from build123d import *

# Parameters (mm, degrees)
BOSS_EXTRUDE1_START     = -2.5
BOSS_EXTRUDE1_DEPTH     = 26.5
CUT_EXTRUDE1_START      = -3
CUT_EXTRUDE1_DEPTH      = 25.6
CUT_EXTRUDE2_DEPTH      = 53.459508194
CUT_EXTRUDE2_DEPTH_BACK = 53.459508194
SKETCH3_W               = 33
SKETCH3_H               = 5.5
CUT_EXTRUDE3_DEPTH      = 53.459508194
CUT_EXTRUDE3_DEPTH_BACK = 53.459508194
SKETCH4_R               = 1.2


with BuildPart() as part:
    # Sketch1 → Boss-Extrude1 (new body)
    with BuildSketch(Plane.XY.offset(BOSS_EXTRUDE1_START)):
        Polygon((40, 16), (39.846282243, 17.560722576), (39.39103626, 19.061467459), (38.651756898, 20.444561864), (37.656854249, 21.656854249), (36.444561864, 22.651756898), (35.061467459, 23.39103626), (33.560722576, 23.846282243), (32, 24), (-32, 24), (-33.560722576, 23.846282243), (-35.061467459, 23.39103626), (-36.444561864, 22.651756898), (-37.656854249, 21.656854249), (-38.651756898, 20.444561864), (-39.39103626, 19.061467459), (-39.846282243, 17.560722576), (-40, 16), (-40, -16), (-39.846282243, -17.560722576), (-39.39103626, -19.061467459), (-38.651756898, -20.444561864), (-37.656854249, -21.656854249), (-36.444561864, -22.651756898), (-35.061467459, -23.39103626), (-33.560722576, -23.846282243), (-32, -24), (32, -24), (33.560722576, -23.846282243), (35.061467459, -23.39103626), (36.444561864, -22.651756898), (37.656854249, -21.656854249), (38.651756898, -20.444561864), (39.39103626, -19.061467459), (39.846282243, -17.560722576), (40, -16), align=None)
    extrude(amount=BOSS_EXTRUDE1_DEPTH)

    # Sketch2 → Cut-Extrude1 (cut)
    with BuildSketch(Plane.XY.offset(CUT_EXTRUDE1_START)):
        Polygon((38.4, 16), (38.277025795, 17.248578061), (37.912829008, 18.449173967), (37.321405519, 19.555649491), (36.5254834, 20.5254834), (35.555649491, 21.321405519), (34.449173967, 21.912829008), (33.248578061, 22.277025795), (32, 22.4), (-32, 22.4), (-33.248578061, 22.277025795), (-34.449173967, 21.912829008), (-35.555649491, 21.321405519), (-36.5254834, 20.5254834), (-37.321405519, 19.555649491), (-37.912829008, 18.449173967), (-38.277025795, 17.248578061), (-38.4, 16), (-38.4, -16), (-38.277025795, -17.248578061), (-37.912829008, -18.449173967), (-37.321405519, -19.555649491), (-36.5254834, -20.5254834), (-35.555649491, -21.321405519), (-34.449173967, -21.912829008), (-33.248578061, -22.277025795), (-32, -22.4), (32, -22.4), (33.248578061, -22.277025795), (34.449173967, -21.912829008), (35.555649491, -21.321405519), (36.5254834, -20.5254834), (37.321405519, -19.555649491), (37.912829008, -18.449173967), (38.277025795, -17.248578061), (38.4, -16), align=None)
    extrude(amount=CUT_EXTRUDE1_DEPTH, mode=Mode.SUBTRACT)

    # Sketch3 → Cut-Extrude2 (cut, two sides: drawn at the far end of the back side and taken through both)
    with BuildSketch(Plane.XY.offset(-CUT_EXTRUDE2_DEPTH_BACK)):
        with Locations((15, 17.725)):
            Rectangle(SKETCH3_W, SKETCH3_H)
        with Locations((-15, -17.725)):
            Rectangle(SKETCH3_W, SKETCH3_H)
    extrude(amount=CUT_EXTRUDE2_DEPTH + CUT_EXTRUDE2_DEPTH_BACK, mode=Mode.SUBTRACT)

    # Sketch4 → Cut-Extrude3 (cut, two sides: drawn at the far end of the back side and taken through both)
    with BuildSketch(Plane.XY.offset(-CUT_EXTRUDE3_DEPTH_BACK)):
        with Locations((30, 0)):
            Circle(SKETCH4_R)
        with Locations((-30, 0)):
            Circle(SKETCH4_R)
    extrude(amount=CUT_EXTRUDE3_DEPTH + CUT_EXTRUDE3_DEPTH_BACK, mode=Mode.SUBTRACT)


solid = part.part
Geometry check sheet. Reference: the model listing, model coordinates, mm. A direction names the side the tool comes from. Round coordinates to 2 decimals unless told otherwise and drop trailing zeros. Order: outer loops, then holes, each group sorted by start corner. A loop starts at its lowest first (then second) coordinate and runs counter-clockwise, first axis right, second up. Notation, with made-up numbers: (-15.75, 13) -> (9.25, 13) arc R27 cw to (9.25, 36) -> close; hole circle Ø9 at (75, -11.75). An arc over 180 degrees is marked (long way). Use one line per item in the form item = value.
1. Mould release check, pull along X, two halves, no side actions. Record for faces 3 (the face through (-34.322, -23.615, 10.564)), 4 (the face through (39.615, -18.322, 10.564)), 5 (the face through (-1, 0, 22.6)): pulls with the +X half, pulls with the -X half, needs draft (parallel to the pull), parting line crosses it, or undercut.
Working result:
face_3 = pulls with the -X half
face_4 = pulls with the +X half
face_5 = undercut
2. Scan lines: line 1 along X through (y, z) = (0, 23.6); line 2 along Y through (x, z) = (30, 23.5) (3 decimals); line 3 along X through (y, z) = (-0.5, 21.5). Record each from-to range of solid material in increasing order. Write a range as from..to.
Working result:
line_1 = -40..-31.2, -28.8..28.8, 31.2..40
line_2 = -24..-1.2, 1.2..14.975, 20.475..24
line_3 = -40..-38.4, 38.4..40
3. Set-up check for faces 1 (the face through (39.922, -16.791, 10.564)), 2 (the face through (38.4, 0, 10)): record each of +Z, -Z, +X, -X, +Y, -Y from which the full face is reachable in a straight line by a thin tool's end or side.
Working result:
face_1 = +Z, -Z, +X, -Y
face_2 = -Z
4. Cross-section at D-D, the plane y = 9.5. Enter the section's corners in (x, z).
Working result:
outline = (-40, -2.5) -> (-38.4, -2.5) -> (-38.4, 22.6) -> (38.4, 22.6) -> (38.4, -2.5) -> (40, -2.5) -> (40, 24) -> (-40, 24) -> close
5. Cross-section at B-B, the plane y = 0. Enter the section's corners in (x, z), plus the area to 3 significant figures.
Working result:
outline = (-40, -2.5) -> (-38.4, -2.5) -> (-38.4, 22.6) -> (-31.2, 22.6) -> (-31.2, 24) -> (-40, 24) -> close; (-28.8, 22.6) -> (28.8, 22.6) -> (28.8, 24) -> (-28.8, 24) -> close; (31.2, 22.6) -> (38.4, 22.6) -> (38.4, -2.5) -> (40, -2.5) -> (40, 24) -> (31.2, 24) -> close
area = 186 mm^2
6. Cross-section at A-A, the plane x = -2.5. Enter the section's corners in (y, z) (3 decimals), plus the area to 3 significant figures.
Working result:
outline = (-24, -2.5) -> (-22.4, -2.5) -> (-22.4, 22.6) -> (-20.475, 22.6) -> (-20.475, 24) -> (-24, 24) -> close; (-14.975, 22.6) -> (22.4, 22.6) -> (22.4, -2.5) -> (24, -2.5) -> (24, 24) -> (-14.975, 24) -> close
area = 140 mm^2
7. Cross-section at C-C, the plane x = 30. Enter the section's corners in (y, z) (3 decimals).
Working result:
outline = (-24, -2.5) -> (-22.4, -2.5) -> (-22.4, 22.6) -> (-1.2, 22.6) -> (-1.2, 24) -> (-24, 24) -> close; (1.2, 22.6) -> (14.975, 22.6) -> (14.975, 24) -> (1.2, 24) -> close; (20.475, 22.6) -> (22.4, 22.6) -> (22.4, -2.5) -> (24, -2.5) -> (24, 24) -> (20.475, 24) -> close
8. Go/stop test with flat-tipped pins: pin 1 (3 mm diameter, centred on x = 19, y = 11.5, fed in from -Z); pin 2 (2 mm diameter, centred on x = 30, y = 0, fed in from -Z); pin 3 (1.5 mm diameter, centred on y = 18.5, z = 23.5, fed in from +X); pin 4 (1.1 mm diameter, centred on y = -18, z = 23.5, fed in from -X). Record where each tip stops, or that it passes through.
Working result:
pin_1 = 22.6
pin_2 = through
pin_3 = 39.79
pin_4 = -39.86
